Drawing for the job (mm, zero at the part's lowest x, y, z). A direction names the side the tool comes from. Round coordinates to 2 decimals unless told otherwise and drop trailing zeros. Loops run counter-clockwise (first coordinate to the right, second up) from the corner with the lowest first, then second, coordinate; pieces in that order, holes last.
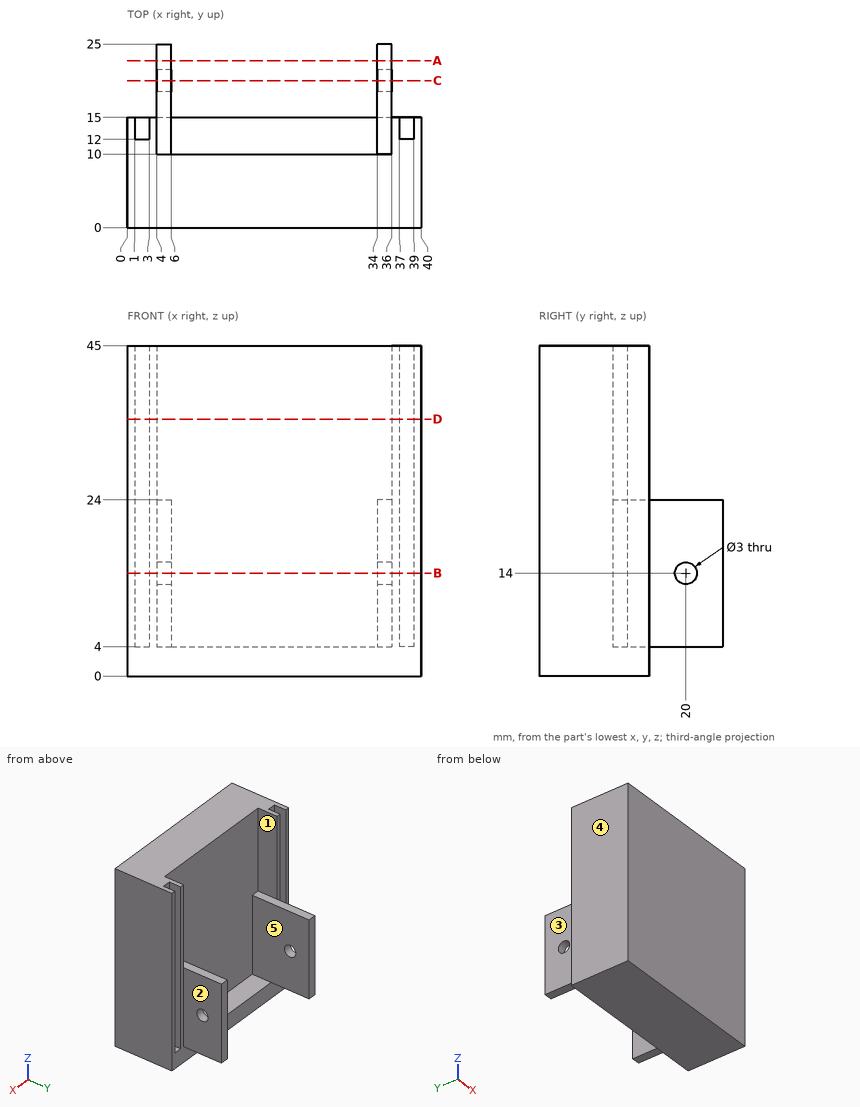
Q1. Slice it at B-B on z = 14. Give the cut face in (x, y).
Q2. Slice it at D-D on z = 35. Give the cut face in (x, y).
Q3. Pull direction X, two halves, no side cores. Call the marked faces 1, 2 and 3: pulls with the +X half, pulls with the -X half, needs draft (parallel to the pull), parting line crosses it, or undercut.
Q4. Slice it at C-C on y = 20. Give the cut face in (x, z).
Q5. Tool access for the marked faces 4 and 5: list every direction of +Z, -Z, +X, -X, +Y, -Y with a clear straight run to the whole face (end or side of a thin tool).
Q6. Flat gauge pins, fed straight in: P1, Ø0.6, axis at x = 4.5, y = 20.5, coming from the -Z side; P2, Ø0.9, axis at y = 13.5, z = 22, coming from the -X side; P3, Ø9.5, axis at x = 15, z = 25.5, coming from the +Y side; P4, Ø1, axis at x = 38, z = 24, coming from the +Y side. Where does each tip first touch, or does it go through?
Q7. Slice it at A-A on y = 22.75. Give the cut face in (x, z).
Q8. Probe line 1 (X direction, y = 13.5, z = 35.5); line 2 (X direction, y = 12.5, z = 9); line 3 (Z direction, x = 4.7, y = 20). List the from-to ranges inside material, lowest first.
Reply:
1. outline: (0, 0) - (40, 0) - (40, 15) - (39, 15) - (39, 12) - (37, 12) - (37, 15) - (36, 15) - (36, 18.5) - (34, 18.5) - (34, 10) - (6, 10) - (6, 18.5) - (4, 18.5) - (4, 15) - (3, 15) - (3, 12) - (1, 12) - (1, 15) - (0, 15) - close; (4, 21.5) - (6, 21.5) - (6, 25) - (4, 25) - close; (34, 21.5) - (36, 21.5) - (36, 25) - (34, 25) - close
2. outline: (0, 0) - (40, 0) - (40, 15) - (39, 15) - (39, 12) - (37, 12) - (37, 15) - (36, 15) - (36, 10) - (4, 10) - (4, 15) - (3, 15) - (3, 12) - (1, 12) - (1, 15) - (0, 15) - close
3. face 1: undercut
3. face 2: pulls with the +X half
3. face 3: pulls with the -X half
4. outline: (4, 4) - (6, 4) - (6, 12.5) - (4, 12.5) - close; (4, 15.5) - (6, 15.5) - (6, 24) - (4, 24) - close; (34, 4) - (36, 4) - (36, 12.5) - (34, 12.5) - close; (34, 15.5) - (36, 15.5) - (36, 24) - (34, 24) - close
5. face 4: +Z, -Z, -X, +Y, -Y
5. face 5: +Z, +Y
6. P1: stops at z = 4
6. P2: stops at x = 0
6. P3: stops at y = 10
6. P4: stops at y = 12
7. outline: (4, 4) - (6, 4) - (6, 24) - (4, 24) - close; (34, 4) - (36, 4) - (36, 24) - (34, 24) - close
8. line 1: x = 0 to 1, 3 to 4, 36 to 37, 39 to 40
8. line 2: x = 0 to 1, 3 to 6, 34 to 37, 39 to 40
8. line 3: z = 4 to 12.5, 15.5 to 24
